Design review of the part shown in the three views and the two pictorial views. Dimensions are in mm from the part's minimum x, y and z. Round coordinates to 2 decimals unless told otherwise and drop trailing zeros. Order: outer loops, then holes, each group sorted by start corner. A loop starts at its lowest first (then second) coordinate and runs counter-clockwise, first axis right, second up.
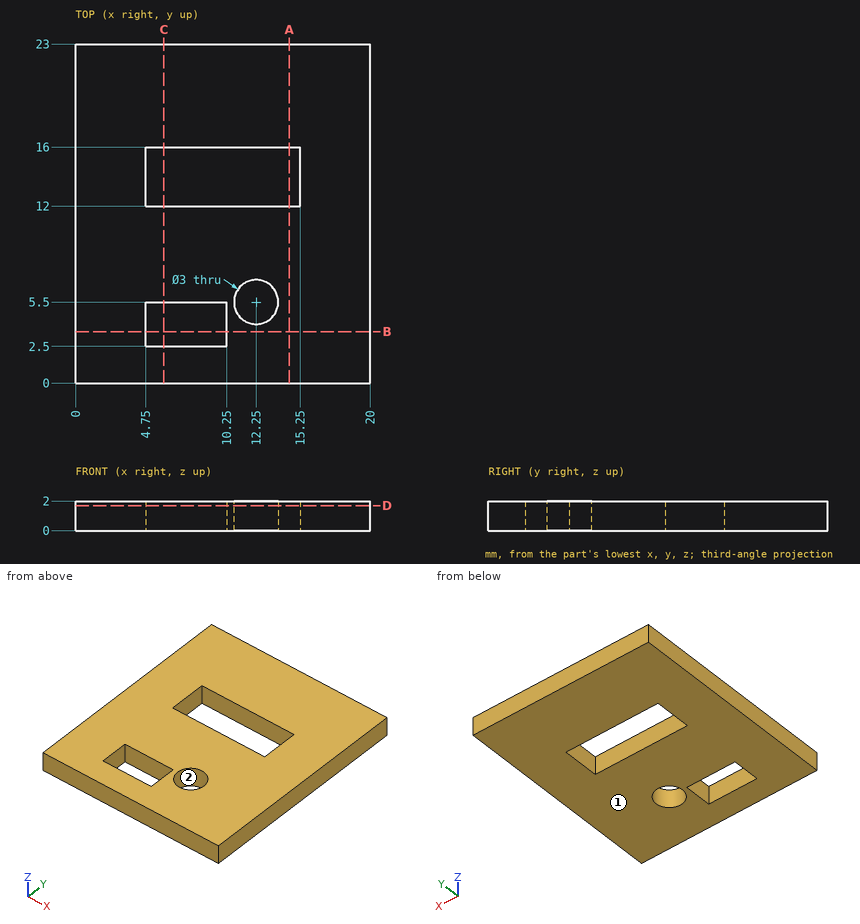
(1) Consider section C-C (x = 6). Write out the cut boundary in (y, z), and give its area (3 significant figures).
Data:
outline: (0, 0) - (2.5, 0) - (2.5, 2) - (0, 2) - close; (5.5, 0) - (12, 0) - (12, 2) - (5.5, 2) - close; (16, 0) - (23, 0) - (23, 2) - (16, 2) - close
area: 32.0 mm2
(2) Consider section D-D (z = 1.7). Write out the cut boundary in (x, y), and give its area (3 significant figures).
Data:
outline: (0, 0) - (20, 0) - (20, 23) - (0, 23) - close; hole (4.75, 2.5) - (10.25, 2.5) - (10.25, 5.5) - (4.75, 5.5) - close; hole (4.75, 12) - (15.25, 12) - (15.25, 16) - (4.75, 16) - close; hole circle Ø3 at (12.25, 5.5)
area: 394 mm2
(3) To check wall thickness, follow probe 1 along Y at (x, z) = (12.25, 0.5); probe 2 along Y at (x, z) = (8, 1.8); probe 3 along Y at (x, z) = (15, 1.7). State the ranges of each line that lie inside material, in increasing order.
Data:
probe 1: y = 0 to 4, 7 to 12, 16 to 23
probe 2: y = 0 to 2.5, 5.5 to 12, 16 to 23
probe 3: y = 0 to 12, 16 to 23
(4) Consider section A-A (x = 14.5). Write out the cut boundary in (y, z).
Data:
outline: (0, 0) - (12, 0) - (12, 2) - (0, 2) - close; (16, 0) - (23, 0) - (23, 2) - (16, 2) - close
(5) Draft analysis for pull direction X (two halves, no side actions). For the marked faces 1 and 2, state which applies: pulls with the +X half, pulls with the -X half, needs draft (parallel to the pull), parting line crosses it, or undercut.
Data:
face 1: needs draft
face 2: undercut
(6) Consider section B-B (y = 3.5). Write out the cut boundary in (x, z), and give its area (3 significant figures).
Data:
outline: (0, 0) - (4.75, 0) - (4.75, 2) - (0, 2) - close; (10.25, 0) - (20, 0) - (20, 2) - (10.25, 2) - close
area: 29.0 mm2
